The listing builds one solid part. Answer for the finished solid, in the listing's coordinates (mm). A direction names the side the tool comes from. Round coordinates to 2 decimals unless told otherwise and drop trailing zeros. Write each loop counter-clockwise with the first axis right and the second up, starting at its lowest first coordinate (ties: lowest second). Pieces come first, ordered by that corner, then holes.
from build123d import *

# Parameters (mm, degrees)
PAD_DEPTH       = 5
SKETCH001_R     = 1.5
POCKET_DEPTH    = 5.001
SKETCH002_R     = 3
POCKET001_DEPTH = 3


with BuildPart() as part:
    # Sketch → Pad (new body)
    with BuildSketch(Plane.XZ):
        Polygon((0, 0), (0, 10), (0.1, 10), (66, 54.75), (76, 54.75), (76, 0), align=None)
    extrude(amount=PAD_DEPTH)

    # Sketch001 (on Face8 of Pad) → Pocket (cut, through all)
    with BuildSketch(Plane.XZ.offset(5)):
        with Locations((5, 5)):
            Circle(SKETCH001_R)
        with Locations((71, 51)):
            Circle(SKETCH001_R)
        with Locations((71, 43.5)):
            Circle(SKETCH001_R)
        with Locations((71, 28.5)):
            Circle(SKETCH001_R)
    extrude(amount=-POCKET_DEPTH, mode=Mode.SUBTRACT)

    # Sketch002 (on Face5 of Pocket) → Pocket001 (cut)
    with BuildSketch(Plane.XZ.offset(5)):
        with Locations((71, 28.5)):
            Circle(SKETCH002_R)
        with Locations((71, 43.5)):
            Circle(SKETCH002_R)
        with Locations((71, 51)):
            Circle(SKETCH002_R)
        with Locations((5, 5)):
            Circle(SKETCH002_R)
    extrude(amount=-POCKET001_DEPTH, mode=Mode.SUBTRACT)


solid = part.part
1. Section B-B on y = -1.1 is taken. Determine the outline of the cut face in (x, z), plus the area to 3 significant figures.
Geometry says:
outline: (0, 0) - (76, 0) - (76, 54.75) - (66, 54.75) - (0.1, 10) - (0, 10) - close; hole circle Ø3 at (5, 5); hole circle Ø3 at (71, 28.5); hole circle Ø3 at (71, 43.5); hole circle Ø3 at (71, 51)
area: 2,650 mm2
2. Given pin 1 (1.8 mm diameter, centred on x = 6, z = 5, fed in from -Y); pin 2 (2.5 mm diameter, centred on x = 71, z = 43.5, fed in from +Y), each flat-ended and moving along its own axis, determine where each tip first touches the part or whether it passes through.
Geometry says:
pin 1: stops at y = -2
pin 2: passes through
3. Straight lines are drawn through the part: line 1 along Z through (x, y) = (71, -0.65); line 2 along Z through (x, y) = (71, -2.8); line 3 along Y through (x, z) = (69, 26.5). For each, find the intervals that lie inside material, in ascending order.
Geometry says:
line 1: z = 0 to 27, 30 to 42, 45 to 49.5, 52.5 to 54.75
line 2: z = 0 to 25.5, 31.5 to 40.5, 46.5 to 48, 54 to 54.75
line 3: y = -2 to 0
4. For a pull along X with two mould halves and no side action, classify faces 3 (the face through (68.79, -3.52, 53.03)), 4 (the face through (47, 0, 22)), 5 (the face through (32.589, -2.465, 32.062)) as released by +X, released by -X, zero draft, split by the parting line, or undercut.
Geometry says:
face 3: undercut
face 4: zero draft
face 5: released by -X
5. A tool of negligible diameter and unlimited length cuts with its end or side. For faces 1 (the face through (39, -2, 0)), 2 (the face through (68.79, -3.52, 45.53)), from which of +Z, -Z, +X, -X, +Y, -Y can it reach the whole face along a straight path? Write none if from no direction.
Geometry says:
face 1: -Z, +X, -X, +Y, -Y
face 2: -Y
6. Section C-C on x = 5 is taken. Determine the outline of the cut face in (y, z), plus the area to 3 significant figures.
Geometry says:
outline: (-5, 0) - (0, 0) - (0, 3.5) - (-2, 3.5) - (-2, 2) - (-5, 2) - close; (-5, 8) - (-2, 8) - (-2, 6.5) - (0, 6.5) - (0, 13.33) - (-5, 13.33) - close
area: 42.6 mm2
7. Section A-A on z = 5 is taken. Determine the outline of the cut face in (x, y), plus the area to 3 significant figures.
Geometry says:
outline: (0, -5) - (2, -5) - (2, -2) - (3.5, -2) - (3.5, 0) - (0, 0) - close; (6.5, -2) - (8, -2) - (8, -5) - (76, -5) - (76, 0) - (6.5, 0) - close
area: 356 mm2
8. Section D-D on x = 19 is taken. Determine the outline of the cut face in (y, z), plus the area to 3 significant figures.
Geometry says:
outline: (-5, 0) - (0, 0) - (0, 22.83) - (-5, 22.83) - close
area: 114 mm2
